```python
from build123d import *

# Parameters (mm, degrees)
PAD003_DEPTH  = 7
SKETCH002_R   = 5
PAD002_DEPTH  = 50
SKETCH001_R   = 2.9
SKETCH001_R_2 = 2
PAD001_DEPTH  = 100
PAD_DEPTH     = 20


with BuildPart() as clamp_slot:
    # Sketch003 → Pad003 (new body)
    with BuildSketch(Plane.YZ):
        with BuildLine():
            ThreePointArc((78.5, 10), (66, 16.708438), (53.5, 10))
            Line((53.5, 10), (53.5, 25))
            Line((53.5, 25), (78.5, 25))
            Line((78.5, 25), (78.5, 10))
        make_face()
    extrude(amount=PAD003_DEPTH)


with BuildPart() as screw_recesses:
    # Sketch002 → Pad002 (new body)
    with BuildSketch(Plane.XY.offset(7)):
        with Locations((0, 66)):
            Circle(SKETCH002_R)
        with Locations((70, 8)):
            Circle(SKETCH002_R)
    extrude(amount=PAD002_DEPTH)


with BuildPart() as screw_holes:
    # Sketch001 → Pad001 (new body)
    with BuildSketch(Plane.XY):
        with Locations((70, 65)):
            Circle(SKETCH001_R)
        with Locations((70, 20)):
            Circle(SKETCH001_R)
        with Locations((70, 8)):
            Circle(SKETCH001_R_2)
        with Locations((0, 66)):
            Circle(SKETCH001_R_2)
    extrude(amount=PAD001_DEPTH)


with BuildPart() as cut002:
    # Sketch → Pad (new body)
    with BuildSketch(Plane.XY):
        Polygon((0, 76.12), (80, 76.12), (80, 0), (60, 0), (60, 56.12), (0, 56.12), align=None)
    extrude(amount=PAD_DEPTH)

    # Cut: cut Screw Holes
    add(screw_holes.part, mode=Mode.SUBTRACT)

    # Cut001: cut Screw Recesses
    add(screw_recesses.part, mode=Mode.SUBTRACT)

    # Cut002: cut Clamp Slot
    add(clamp_slot.part, mode=Mode.SUBTRACT)


with BuildPart() as fusion:
    # Part__Mirroring: instance of Cut002
    add(cut002.part.mirror(Plane(origin=(0, 0, 0), x_dir=(0, -1, 0), z_dir=(1, 0, 0))))

    # Fusion: union Cut002
    add(cut002.part)


solid = fusion.part
```
Geometry check sheet. Reference: the model listing, model coordinates, mm. A direction names the side the tool comes from. Coordinates: 2 decimals unless noted, no trailing zeros. Loops run counter-clockwise (first coordinate to the right, second up) from the corner with the lowest first, then second, coordinate; pieces in that order, holes last. Notation, with made-up numbers: (-5.75, 75.25) - (20.25, 75.25) arc R13 ccw to (20.25, 82.25) - close; hole circle Ø7 at (23, -28). An arc over 180 degrees is marked (long way). One line per item, written item: value. Start each with the question number.
(1) Tool access check on faces 1 (the cylindrical face through (0, 61, 12)), 2 (the flat face through (1, 56.12, 10)), 3 (the cylindrical face through (-71.908, 8.601, 3.451)). Record the directions out of +Z, -Z, +X, -X, +Y, -Y that give a thin tool (end or side, any length) a straight path to the whole face; none if there is none.
(2) Cross-section at B-B on z = 10.5. Enter the section's corners in (x, y).
(3) Material ranges on line 1 (X direction, y = 8, z = 15.75); line 2 (Y direction, x = -70, z = 4.5); line 3 (Y direction, x = -70, z = 14), recorded low to high. Write a range as [from, to].
(4) Cross-section at C-C on y = 47. Enter the section's corners in (x, z).
(5) Mould release check, pull along X, two halves, no side actions. Record for faces 4 (the flat face through (60.2, 47.1, 20)), 5 (the flat face through (-60, 28, 10)), 6 (the flat face through (80, 39, 10)): released by +X, released by -X, zero draft, split by the parting line, or undercut.
(6) Cross-section at D-D on y = 8. Enter the section's corners in (x, z).
(7) Cross-section at A-A on x = 70. Enter the section's corners in (y, z).
(8) Depth check by flat-ended pin: P1, Ø4.5, axis at x = 0, y = 66, coming from the +Z side. Enter the tip coordinate at first touch or a pass-through.
Results below:
1. face 1: +Z
1. face 2: +Z, -Z, -Y
1. face 3: +Z, -Z
2. outline: (-80, 0) - (-60, 0) - (-60, 56.12) - (60, 56.12) - (60, 0) - (80, 0) - (80, 76.12) - (-80, 76.12) - close; hole circle Ø10 at (-70, 8); hole circle Ø5.8 at (-70, 20); hole circle Ø5.8 at (-70, 65); hole circle Ø10 at (0, 66); hole circle Ø10 at (70, 8); hole circle Ø5.8 at (70, 20); hole circle Ø5.8 at (70, 65)
3. line 1: x = [-80, -75], [-65, -60], [60, 65], [75, 80]
3. line 2: y = [0, 6], [10, 17.1], [22.9, 62.1], [67.9, 76.12]
3. line 3: y = [0, 3], [13, 17.1], [22.9, 62.1], [67.9, 76.12]
4. outline: (-80, 0) - (-60, 0) - (-60, 20) - (-80, 20) - close; (60, 0) - (80, 0) - (80, 20) - (60, 20) - close
5. face 4: zero draft
5. face 5: undercut
5. face 6: released by +X
6. outline: (-80, 0) - (-72, 0) - (-72, 7) - (-75, 7) - (-75, 20) - (-80, 20) - close; (-68, 0) - (-60, 0) - (-60, 20) - (-65, 20) - (-65, 7) - (-68, 7) - close; (60, 0) - (68, 0) - (68, 7) - (65, 7) - (65, 20) - (60, 20) - close; (72, 0) - (80, 0) - (80, 20) - (75, 20) - (75, 7) - (72, 7) - close
7. outline: (0, 0) - (6, 0) - (6, 7) - (3, 7) - (3, 20) - (0, 20) - close; (10, 0) - (17.1, 0) - (17.1, 20) - (13, 20) - (13, 7) - (10, 7) - close; (22.9, 0) - (62.1, 0) - (62.1, 20) - (22.9, 20) - close; (67.9, 0) - (76.12, 0) - (76.12, 20) - (67.9, 20) - close
8. P1: stops at z = 7
